Part model, mm, in its own coordinate system. Face numbers are marked on the shaded views. A direction names the side the tool comes from. Give positions to 0.01 mm unless a question says otherwise; leave off trailing zeros. Order: outer loops, then holes, each group sorted by start corner. A loop starts at its lowest first (then second) coordinate and runs counter-clockwise, first axis right, second up. Notation, with made-up numbers: (85.5, -38) - (108.5, -38) arc R21 cw to (108.5, -22) - close; hole circle Ø11 at (30.25, -38.75). An arc over 180 degrees is marked (long way). One line per item, written item: value.
```python
from build123d import *

# Parameters (mm, degrees)
BOSS_EXTRUDE1_DEPTH = 35
SKETCH2_R           = 10
BOSS_EXTRUDE2_DEPTH = 20
FILLET1_R           = 1.5
FILLET2_R           = 1.5


with BuildPart() as part:
    # Sketch1 → Boss-Extrude1 (new body, symmetric)
    with BuildSketch(Plane.XY):
        Polygon((0, 0), (0, 20), (15, 20), (15, 40), (35, 40), (35, 20), (50, 20), (50, 0), align=None)
    extrude(amount=BOSS_EXTRUDE1_DEPTH, both=True)

    # Sketch2 → Boss-Extrude2 (add)
    with BuildSketch(Plane(origin=(0, 0, 0), x_dir=(-1, 0, 0), z_dir=(0, -1, 0))):
        with Locations((-25, 0)):
            Circle(SKETCH2_R)
    extrude(amount=BOSS_EXTRUDE2_DEPTH)

    # Fillet1
    fillet1_edges = [part.edges().sort_by_distance(p)[0] for p in [
        (35, 30, -35),
        (42.5, 20, -35),
        (50, 10, -35),
        (25, 0, -35),
        (42.5, 20, 35),
        (0, 0, 0),
        (0, 20, 0),
        (15, 20, 0),
        (15, 40, 0),
        (35, 40, 0),
        (35, 20, 0),
        (50, 20, 0),
        (50, 0, 0),
        (35, 30, 35),
        (25, 40, 35),
        (35, 0, 0),
        (15, 30, 35),
        (7.5, 20, 35),
        (0, 10, 35),
        (25, 0, 35),
        (0, 10, -35),
        (50, 10, 35),
        (7.5, 20, -35),
        (15, 30, -35),
        (25, 40, -35),
    ]]
    fillet(fillet1_edges, radius=FILLET1_R)

    # Fillet2
    fillet2_edges = [part.edges().sort_by_distance(p)[0] for p in [
        (35, -20, 0),
    ]]
    fillet(fillet2_edges, radius=FILLET2_R)


solid = part.part
```
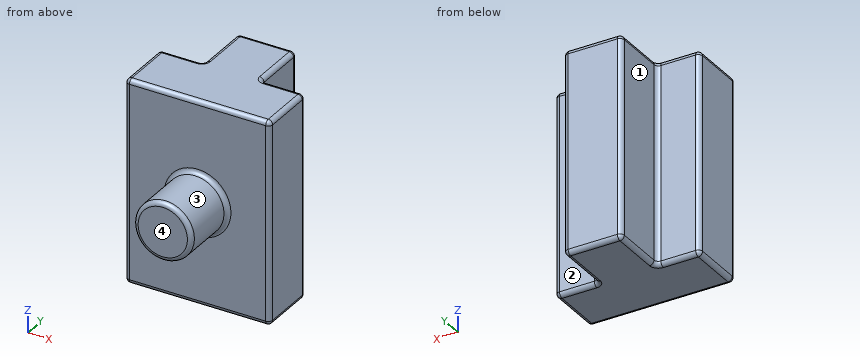
1) Slice it at C-C on z = 0. Write the cut outline in (x, y), then the cut area to 3 significant figures.
Answer:
outline: (0, 1.5) arc R1.5 ccw to (1.5, 0) - (13.5, 0) arc R1.5 cw to (15, -1.5) - (15, -18.5) arc R1.5 ccw to (16.5, -20) - (33.5, -20) arc R1.5 ccw to (35, -18.5) - (35, -1.5) arc R1.5 cw to (36.5, 0) - (48.5, 0) arc R1.5 ccw to (50, 1.5) - (50, 18.5) arc R1.5 ccw to (48.5, 20) - (36.5, 20) arc R1.5 cw to (35, 21.5) - (35, 38.5) arc R1.5 ccw to (33.5, 40) - (16.5, 40) arc R1.5 ccw to (15, 38.5) - (15, 21.5) arc R1.5 cw to (13.5, 20) - (1.5, 20) arc R1.5 ccw to (0, 18.5) - close
area: 1,800 mm2
2) Drop flat-ended pins along their axis: P1, Ø8.5, axis at y = 28, z = -8.5, coming from the -X side; P2, Ø5, axis at y = 27, z = 6, coming from the +X side; P3, Ø9.5, axis at x = 9.5, z = 10.5, coming from the +Y side. Give the stop position or say it passes through.
Answer:
P1: stops at x = 15
P2: stops at x = 35
P3: stops at y = 20.2
3) Slice it at D-D on y = -10.5. Write the cut outline in (x, z), then the cut area to 3 significant figures.
Answer:
outline: circle Ø20 at (25, 0)
area: 314 mm2
4) Slice it at A-A on z = 13.5. Write the cut outline in (x, y), then the cut area to 3 significant figures.
Answer:
outline: (0, 1.5) arc R1.5 ccw to (1.5, 0) - (48.5, 0) arc R1.5 ccw to (50, 1.5) - (50, 18.5) arc R1.5 ccw to (48.5, 20) - (36.5, 20) arc R1.5 cw to (35, 21.5) - (35, 38.5) arc R1.5 ccw to (33.5, 40) - (16.5, 40) arc R1.5 ccw to (15, 38.5) - (15, 21.5) arc R1.5 cw to (13.5, 20) - (1.5, 20) arc R1.5 ccw to (0, 18.5) - close
area: 1,400 mm2
5) Wall check: line 1 along Y through (x, z) = (44, -8); line 2 along X through (y, z) = (29, 6.5); line 3 along Y through (x, z) = (31, -30). Give the ranges that are in metal, low to high. Write a range as [from, to].
Answer:
line 1: y = [0, 20]
line 2: x = [15, 35]
line 3: y = [0, 40]
6) Which spindle directions (+Z, -Z, +X, -X, +Y, -Y) get a long thin tool onto all of the face, cutting with end or side? Do the marked faces 1, 2, 3 and 4. Say none if no direction does.
Answer:
face 1: +Z, -Z, -X, +Y
face 2: +Z, -Z, +X, +Y
face 3: -Y
face 4: +Z, -Z, +X, -X, -Y
7) Slice it at B-B on x = 25. Write the cut outline in (y, z), then the cut area to 3 significant figures.
Answer:
outline: (-20, -8.5) arc R1.5 ccw to (-18.5, -10) - (-1.5, -10) arc R1.5 cw to (0, -11.5) - (0, -33.5) arc R1.5 ccw to (1.5, -35) - (38.5, -35) arc R1.5 ccw to (40, -33.5) - (40, 33.5) arc R1.5 ccw to (38.5, 35) - (1.5, 35) arc R1.5 ccw to (0, 33.5) - (0, 11.5) arc R1.5 cw to (-1.5, 10) - (-18.5, 10) arc R1.5 ccw to (-20, 8.5) - close
area: 3,200 mm2
